Autodesk Inventor part; units mm, degrees
ref_plane "YZ Plane" through (0, 0, 0) normal (1, 0, 0) x (0, 1, 0)
ref_plane "XZ Plane" through (0, 0, 0) normal (0, 1, 0) x (-1, 0, 0)
ref_plane "XY Plane" through (0, 0, 0) normal (0, 0, 1) x (1, 0, 0)
sketch "Skizze1" plane through (0, 0, 0) normal (0, 1, 0) x (-1, 0, 0)
  line L0 (-12.5, 12.5) -> (12.5, 12.5)
  line L1 (12.5, 12.5) -> (12.5, -12.5)
  line L2 (12.5, -12.5) -> (-12.5, -12.5)
  line L3 (-12.5, -12.5) -> (-12.5, 12.5)
  line L4 (-12.5, 12.5) -> (12.5, -12.5) construction
  line L5 (12.5, 12.5) -> (-12.5, -12.5) construction
  line L6 (10, 10) -> (1.5, 10)
  line L7 (1.5, 10) -> (1.5, 1.5)
  line L8 (1.5, 1.5) -> (10, 1.5)
  line L9 (10, 1.5) -> (10, 10)
  line L10 (10, -10) -> (1.5, -10)
  line L11 (1.5, -10) -> (1.5, -1.5)
  line L12 (1.5, -1.5) -> (10, -1.5)
  line L13 (10, -1.5) -> (10, -10)
  line L14 (-1.5, 1.5) -> (-10, 1.5)
  line L15 (-10, 1.5) -> (-10, 10)
  line L16 (-10, 10) -> (-1.5, 10)
  line L17 (-1.5, 10) -> (-1.5, 1.5)
  line L18 (-1.5, -1.5) -> (-10, -1.5)
  line L19 (-10, -1.5) -> (-10, -10)
  line L20 (-10, -10) -> (-1.5, -10)
  line L21 (-1.5, -10) -> (-1.5, -1.5)
  point P0 (0, 0)
  dimension "d0" = 25
  dimension "d1" = 25
  dimension "d2" = 8.5
  dimension "d3" = 8.5
  dimension "d4" = 8.5
  dimension "d5" = 8.5
  dimension "d6" = 8.5
  dimension "d7" = 8.5
  dimension "d8" = 8.5
  dimension "d9" = 8.5
  dimension "d10" = 2.5
  dimension "d11" = 2.5
  dimension "d12" = 2.5
extrude "Extrusion1" add sketch "Skizze1" along normal blind 5
properties part number "Hydrogel_Test"
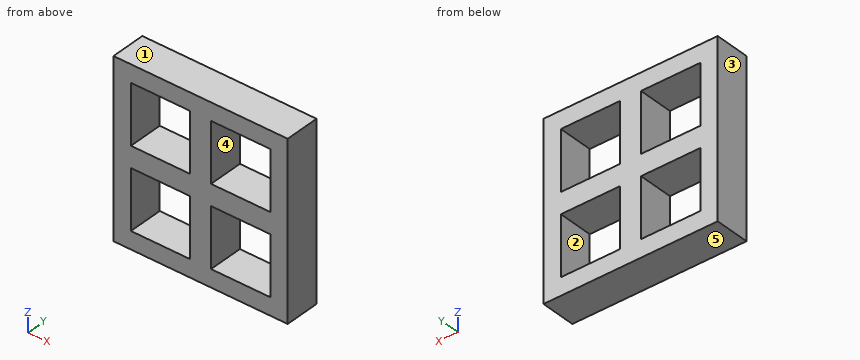
Can you work these out from the model? Positions are in its coordinate system, mm. Face numbers are marked on the shaded views. A direction names the side the tool comes from. Coordinates: 2 decimals unless noted, no trailing zeros. Write each loop counter-clockwise with the first axis right and the second up, starting at its lowest first coordinate (ties: lowest second). Pieces come first, ordered by that corner, then holes. Notation, with made-up numbers: (50.5, 76.5) -> (101.5, 76.5) arc R26 cw to (101.5, 96.5) -> close; hole circle Ø10 at (18.25, -18.75). An arc over 180 degrees is marked (long way). Answer as CSV lines item,"result".
1) If we section it at C-C on y = 4.3: Please give me the cut outline in (x, z).
Check result:
outline,"(-12.5, -12.5) -> (12.5, -12.5) -> (12.5, 12.5) -> (-12.5, 12.5) -> close; hole (-10, -10) -> (-1.5, -10) -> (-1.5, -1.5) -> (-10, -1.5) -> close; hole (-10, 1.5) -> (-1.5, 1.5) -> (-1.5, 10) -> (-10, 10) -> close; hole (1.5, -10) -> (10, -10) -> (10, -1.5) -> (1.5, -1.5) -> close; hole (1.5, 1.5) -> (10, 1.5) -> (10, 10) -> (1.5, 10) -> close"
2) If I drill on line 1 (X direction, y = 3.65, z = 2.5), over which ranges is the centre line in solid material (lowest first)? Write a range as from..to.
Check result:
line 1,"-12.5..-10, -1.5..1.5, 10..12.5"
3) If we section it at B-B on x = -2: Please give me the cut outline in (y, z), then the cut area to 3 significant figures.
Check result:
outline,"(0, -12.5) -> (5, -12.5) -> (5, -10) -> (0, -10) -> close; (0, -1.5) -> (5, -1.5) -> (5, 1.5) -> (0, 1.5) -> close; (0, 10) -> (5, 10) -> (5, 12.5) -> (0, 12.5) -> close"
area,"40.0 mm²"
4) On a 3-axis mill with a long thin cutter (end or side, diameter ignored), from which of +Z, -Z, +X, -X, +Y, -Y can I reach the whole of each face in a straight line? I mean the marked faces 4 and 5. Say none if no direction works.
Check result:
face 4,"+Y, -Y"
face 5,"-Z, +X, -X, +Y, -Y"
5) If we mould it in two halves opening along X, with no side actions, what happens to the marked faces 1, 2 and 3? For each: +X half, -X half, draft (parallel to the pull), parting line (faces both ways), or undercut.
Check result:
face 1,"draft"
face 2,"undercut"
face 3,"-X half"
6) If we section it at A-A on z = 4: Please give me the cut outline in (x, y), then the cut area to 3 significant figures.
Check result:
outline,"(-12.5, 0) -> (-10, 0) -> (-10, 5) -> (-12.5, 5) -> close; (-1.5, 0) -> (1.5, 0) -> (1.5, 5) -> (-1.5, 5) -> close; (10, 0) -> (12.5, 0) -> (12.5, 5) -> (10, 5) -> close"
area,"40.0 mm²"
7) Will this pin go through, and if not, where does the flat tip stop? P1, Ø1.5, axis at x = 7.5, z = -9.5, coming from the +Y side.
Check result:
P1,"y = 5"
